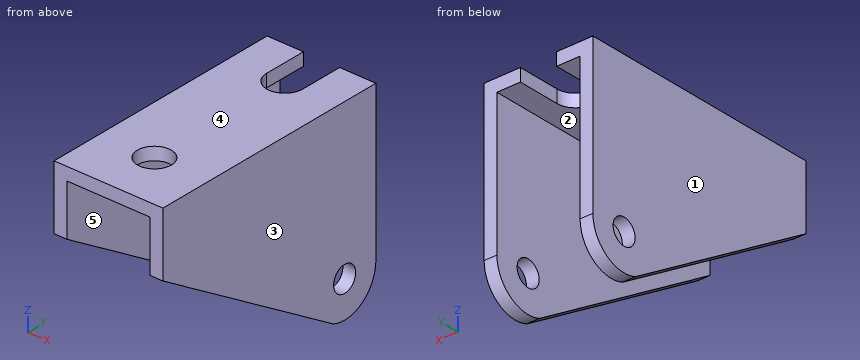
from build123d import *

# Parameters (mm, degrees)
SKETCH012_R             = 3
PAD007_DEPTH            = 12.75
SKETCH013_W             = 45
SKETCH013_H             = 19.5
POCKET004_DEPTH         = 58.001
SKETCH014_R             = 4
POCKET005_DEPTH         = 3.001
BODY003_ROLL_ANGLE      = 180
BODY003_PLACEMENT_ANGLE = -90


with BuildPart() as part:
    # Sketch012 → Pad007 (new body, symmetric)
    with BuildSketch(Plane.XZ):
        with BuildLine():
            Line((-8.5, 0), (-8.5, -36.5))
            Line((-8.5, -36.5), (49.5, -36.5))
            Line((49.5, -36.5), (49.5, -21.5))
            Line((49.5, -21.5), (3.040993, 7.937403))
            ThreePointArc((3.040993, 7.937403), (-4.816719, 7.003515), (-8.5, 0))
        make_face()
        Circle(SKETCH012_R, mode=Mode.SUBTRACT)
    extrude(amount=PAD007_DEPTH, both=True)

    # Sketch013 (on Face1 of Pad007) → Pocket004 (cut, through all)
    with BuildSketch(Plane(origin=(-8.5, 0, 0), x_dir=(0, 0, -1), z_dir=(-1, 0, 0))):
        with Locations((11, 0)):
            Rectangle(SKETCH013_W, SKETCH013_H)
    extrude(amount=-POCKET004_DEPTH, mode=Mode.SUBTRACT)

    # Sketch014 (on Face7 of Pocket004) → Pocket005 (cut, through all)
    with BuildSketch(Plane(origin=(0, 0, -33.5), x_dir=(-1, 0, 0), z_dir=(0, 0, 1))):
        with Locations((-37, 0)):
            Circle(SKETCH014_R)
        with BuildLine():
            Line((-1.5, 4.25), (8.5, 4.25))
            Line((8.5, 4.25), (8.5, -4.25))
            Line((-1.5, -4.25), (8.5, -4.25))
            ThreePointArc((-1.5, 4.25), (-5.75, 0), (-1.5, -4.25))
        make_face()
    extrude(amount=-POCKET005_DEPTH, mode=Mode.SUBTRACT)


with BuildPart() as part_1:
    # Body003 roll: moved
    add(part.part.rotate(Axis((0, 0, 0), (1, 0, 0)), BODY003_ROLL_ANGLE))


with BuildPart() as part_2:
    # Body003 placement: moved
    add(part_1.part.moved(Location((0, 0, 536))).rotate(Axis((0, 0, 536), (0, 0, 1)), BODY003_PLACEMENT_ANGLE))


solid = part_2.part
The listing builds one solid part. Answer for the finished solid, in the listing's coordinates (mm). Face numbers are marked on the shaded views. A direction names the side the tool comes from. Coordinates: 2 decimals unless noted, no trailing zeros. Order: outer loops, then holes, each group sorted by start corner. A loop starts at its lowest first (then second) coordinate and runs counter-clockwise, first axis right, second up. Notation, with made-up numbers: M 14.25,59 L 56.25,59 A20 ccw 56.25,64 Z; hole C 3,51 d5. An arc over 180 degrees is marked long. Use CSV: the item, a comma, the result in double quotes.
Q1. Straight lines are drawn through the part: L1, parallel to X at y = -9, z = 535; L2, parallel to Z at x = 12, y = 0. For each, find the intervals that lie inside material, in ascending order.
Here are the results:
L1,"-12.75 to -9.75, 9.75 to 12.75"
L2,"527.5 to 533, 539 to 572.5"
Q2. Section D-D (z = 534) is taken. Determine the outline of the cut face in (x, y).
Here are the results:
outline,"M -12.75,-12.41 L -9.75,-12.41 L -9.75,-2.24 L -12.75,-2.24 Z; M -12.75,2.24 L -9.75,2.24 L -9.75,8.26 L -12.75,8.26 Z; M 9.75,-12.41 L 12.75,-12.41 L 12.75,-2.24 L 9.75,-2.24 Z; M 9.75,2.24 L 12.75,2.24 L 12.75,8.26 L 9.75,8.26 Z"
Q3. Section A-A (z = 563.5) is taken. Determine the outline of the cut face in (x, y), then the cut area to 3 significant figures.
Here are the results:
outline,"M -12.75,-49.5 L -9.75,-49.5 L -9.75,8.5 L -12.75,8.5 Z; M 9.75,-49.5 L 12.75,-49.5 L 12.75,8.5 L 9.75,8.5 Z"
area,"348 mm2"
Q4. A tool of negligible diameter and unlimited length cuts with its end or side. For the marked faces 4 and 5, from which of +Z, -Z, +X, -X, +Y, -Y can it reach the whole face along a straight path? Write none if from no direction.
Here are the results:
face 4,"+Z, +X, -X, +Y, -Y"
face 5,"-Z, +Y, -Y"
Q5. Given pin 1 Ø3 at (x, y) = (-9, -27.5) entering from -Z; pin 2 Ø1 at (x, y) = (-6, -16.5) entering from -Z, each flat-ended and moving along its own axis, determine where each tip first touches the part or whether it passes through.
Here are the results:
pin 1,"z = 542.74"
pin 2,"z = 569.5"
Q6. Section C-C (y = -37) is taken. Determine the outline of the cut face in (x, z), then the cut area to 3 significant figures.
Here are the results:
outline,"M -12.75,549.58 L -9.75,549.58 L -9.75,569.5 L -4,569.5 L -4,572.5 L -12.75,572.5 Z; M 4,569.5 L 9.75,569.5 L 9.75,549.58 L 12.75,549.58 L 12.75,572.5 L 4,572.5 Z"
area,"172 mm2"
Q7. Determine the mould class of the marked faces 1, 2 and 3 for opening direction X: pulls with the +X half, pulls with the -X half, needs draft (parallel to the pull), parting line crosses it, or undercut.
Here are the results:
face 1,"pulls with the -X half"
face 2,"undercut"
face 3,"pulls with the +X half"
Q8. Section B-B (y = 0) is taken. Determine the outline of the cut face in (x, z).
Here are the results:
outline,"M -12.75,527.5 L -9.75,527.5 L -9.75,533 L -12.75,533 Z; M -12.75,539 L -9.75,539 L -9.75,569.5 L -4.25,569.5 L -4.25,572.5 L -12.75,572.5 Z; M 4.25,569.5 L 9.75,569.5 L 9.75,539 L 12.75,539 L 12.75,572.5 L 4.25,572.5 Z; M 9.75,527.5 L 12.75,527.5 L 12.75,533 L 9.75,533 Z"
